The figure shows three views and two pictorial views of one solid part (mm, origin at its lowest corner). Answer the questions. A direction names the side the tool comes from. Coordinates: 2 decimals unless noted, no trailing zeros. Order: outer loops, then holes, each group sorted by start corner. A loop starts at its lowest first (then second) coordinate and runs counter-clockwise, first axis right, second up. Notation, with made-up numbers: (45, 35) -> (68, 35) arc R17 ccw to (68, 53) -> close; hole circle Ø2 at (88, 44). An arc over 180 degrees is marked (long way). Write item = value, one per line. Start each with the question number.
Q1. Straight lines are drawn through the part: L1, parallel to Z at x = 44.45, y = 55.75; L2, parallel to Y at x = 5, z = 17.78; L3, parallel to Y at x = 3, z = 109. For each, find the intervals that lie inside material, in ascending order. Write a range as from..to.
Q2. The part is cut by section D-D, the plane y = 34.5. Determine the outline of the cut face in (x, z).
Q3. The part is cut by section A-A, the plane x = 44.45. Determine the outline of the cut face in (y, z), plus the area to 3 significant figures.
Q4. The part is cut by section C-C, the plane z = 104. Determine the outline of the cut face in (x, y), plus the area to 3 significant figures.
Q5. The part is cut by section B-B, the plane y = 15.24. Determine the outline of the cut face in (x, z).
Q6. Which of the six approach directions +Z, -Z, +X, -X, +Y, -Y give full straight-line access (tool end or side, diameter ignored) to the marked faces 1, 2 and 3?
Q7. Flat-ended cylindrical pins translate along their axes: pin 1 (6.5 mm diameter, centred on y = 40.64, z = 17.78, fed in from +X); pin 2 (5 mm diameter, centred on x = 20, y = 41, fed in from +Z); pin 3 (1.5 mm diameter, centred on x = 34.5, y = 18, fed in from -Z). Find the tip coordinate at first contact, or state that the pin passes through.
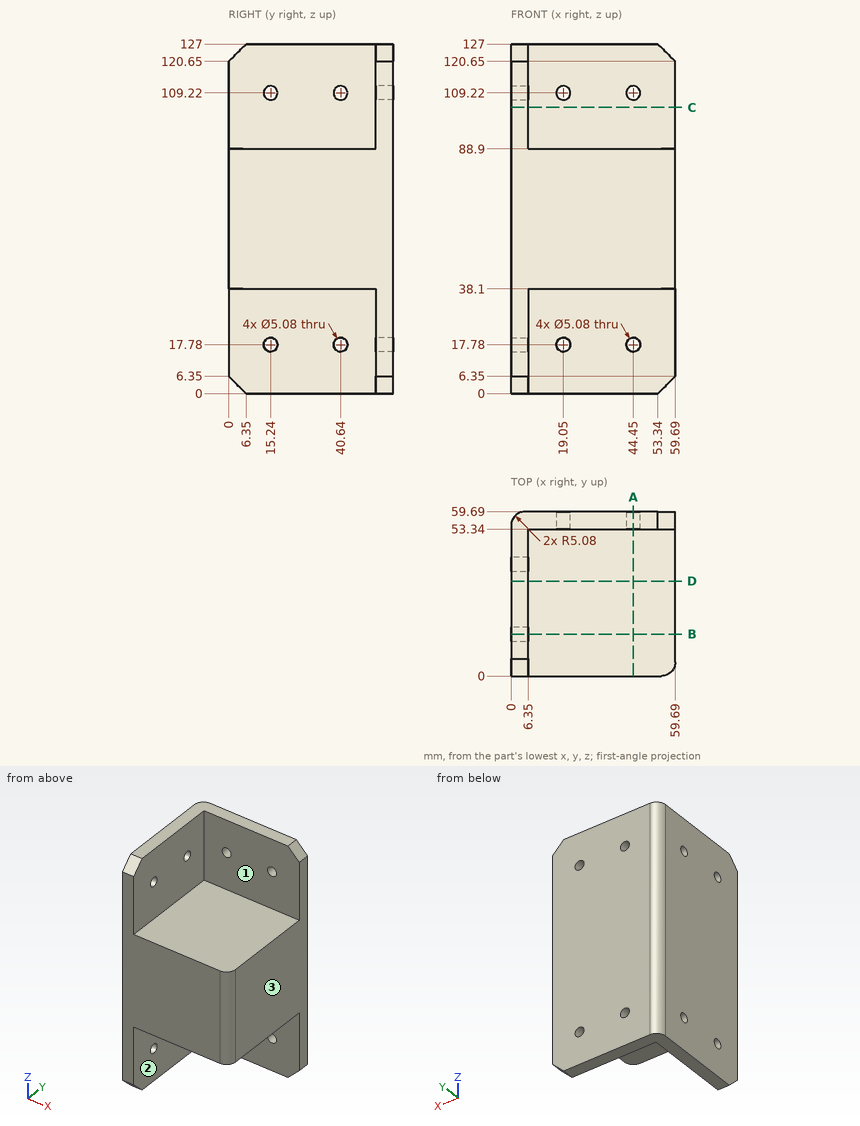
Model answer:
q1.L1 = 0..15.24, 20.32..106.68, 111.76..127
q1.L2 = 0..12.7, 17.78..38.1, 43.18..59.69
q1.L3 = 0..12.71, 17.77..38.11, 43.17..59.24
q2.outline = (0, 0) -> (6.35, 0) -> (6.35, 38.1) -> (59.69, 38.1) -> (59.69, 88.9) -> (6.35, 88.9) -> (6.35, 127) -> (0, 127) -> close
q3.outline = (0, 38.1) -> (53.34, 38.1) -> (53.34, 20.32) -> (59.69, 20.32) -> (59.69, 106.68) -> (53.34, 106.68) -> (53.34, 88.9) -> (0, 88.9) -> close; (53.34, 0) -> (59.69, 0) -> (59.69, 15.24) -> (53.34, 15.24) -> close; (53.34, 111.76) -> (59.69, 111.76) -> (59.69, 127) -> (53.34, 127) -> close
q3.area = 3,450 mm2
q4.outline = (0, 0) -> (6.35, 0) -> (6.35, 53.34) -> (59.69, 53.34) -> (59.69, 59.69) -> (5.08, 59.69) arc R5.08 ccw to (0, 54.61) -> close
q4.area = 712 mm2
q5.outline = (0, 0) -> (6.35, 0) -> (6.35, 15.24) -> (0, 15.24) -> close; (0, 20.32) -> (6.35, 20.32) -> (6.35, 38.1) -> (59.69, 38.1) -> (59.69, 88.9) -> (6.35, 88.9) -> (6.35, 106.68) -> (0, 106.68) -> close; (0, 111.76) -> (6.35, 111.76) -> (6.35, 127) -> (0, 127) -> close
q6.face_1 = +Z, +X, -Y
q6.face_2 = -Z, +X, -Y
q6.face_3 = +Z, -Z, +X, +Y, -Y
q7.pin_1 = 6.35
q7.pin_2 = 88.9
q7.pin_3 = 38.1
